Design review of the part built by this model. Coordinates are the model's own, in mm. A direction names the side the tool comes from. Round coordinates to 2 decimals unless told otherwise and drop trailing zeros. Order: outer loops, then holes, each group sorted by start corner. A loop starts at its lowest first (then second) coordinate and runs counter-clockwise, first axis right, second up. Notation, with made-up numbers: (-29.75, 74) - (-18.75, 74) arc R25 cw to (-18.75, 100) - close; hole circle Ø11 at (53.5, 49.25). An arc over 180 degrees is marked (long way). Answer as a JSON object with one key per item and string values. Group by question number.
from build123d import *

# Parameters (mm, degrees)
F0_R     = 2.13
F1_DEPTH = 5.5


# Not quite as in the source:
# - ends of sketch curves that miss each other by under 0.0002 mm in the source are joined


with BuildPart() as f1:
    # F0 (on Top) → F1 (new body)
    with BuildSketch(Plane.XY):
        with BuildLine():
            ThreePointArc((9.1999998704, 10.271), (8.8197324019, 8.3578320272), (7.735999997, 6.736000003))
            Line((7.735999997, 6.736000003), (-18.536, -19.536))
            ThreePointArc((-18.536, -19.536), (-20.1578320272, -20.6197324019), (-22.071, -20.9999998704))
            Line((-22.071, -20.9999998704), (-46, -21))
            ThreePointArc((-46, -21), (-49.5349996687, -22.4650003313), (-50.9999996674, -26.0000000001))
            Line((-50.9999996674, -26.0000000001), (-51, -37))
            ThreePointArc((-51, -37), (-49.5349996687, -40.5349996687), (-45.9999999999, -41.9999996674))
            Line((-45.9999999999, -41.9999996674), (46, -42))
            ThreePointArc((46, -42), (49.5349996687, -40.5349996687), (50.9999996674, -36.9999999999))
            Line((50.9999996674, -36.9999999999), (51, 37))
            ThreePointArc((51, 37), (49.5349996687, 40.5349996687), (45.9999999999, 41.9999996674))
            Line((45.9999999999, 41.9999996674), (14.2, 42))
            ThreePointArc((14.2, 42), (10.6650003313, 40.5349996687), (9.2000003326, 36.9999999999))
            Line((9.2000003326, 36.9999999999), (9.1999998704, 10.271))
        make_face()
        with Locations((-41.17, -33.07)):
            Circle(F0_R, mode=Mode.SUBTRACT)
        with Locations((-0.17, -33.07)):
            Circle(F0_R, mode=Mode.SUBTRACT)
        with Locations((41.17, -33.07)):
            Circle(F0_R, mode=Mode.SUBTRACT)
        with BuildLine():
            ThreePointArc((13, 4.6), (14.6, 6.2), (16.2, 4.6))
            Line((16.2, 4.6), (16.2, -1.4))
            ThreePointArc((16.2, -1.4), (14.6, -3), (13, -1.4))
            Line((13, -1.4), (13, 4.6))
        make_face(mode=Mode.SUBTRACT)
        with BuildLine():
            Line((47.2, 4.6), (47.2, -1.4))
            ThreePointArc((47.2, -1.4), (45.6, -3), (44, -1.4))
            Line((44, -1.4), (44, 4.6))
            ThreePointArc((44, 4.6), (45.6, 6.2), (47.2, 4.6))
        make_face(mode=Mode.SUBTRACT)
        with BuildLine():
            ThreePointArc((41.6, 14.3), (30.1, 2.8), (18.6, 14.3))
            Line((18.6, 14.3), (18.6, 20.3))
            ThreePointArc((18.6, 20.3), (30.1, 31.8), (41.6, 20.3))
            Line((41.6, 20.3), (41.6, 14.3))
        make_face(mode=Mode.SUBTRACT)
        with BuildLine():
            ThreePointArc((13, 35.6), (14.6, 37.2), (16.2, 35.6))
            Line((16.2, 35.6), (16.2, 29.6))
            ThreePointArc((16.2, 29.6), (14.6, 28), (13, 29.6))
            Line((13, 29.6), (13, 35.6))
        make_face(mode=Mode.SUBTRACT)
        with BuildLine():
            Line((47.2, 35.6), (47.2, 29.6))
            ThreePointArc((47.2, 29.6), (45.6, 28), (44, 29.6))
            Line((44, 29.6), (44, 35.6))
            ThreePointArc((44, 35.6), (45.6, 37.2), (47.2, 35.6))
        make_face(mode=Mode.SUBTRACT)
    extrude(amount=F1_DEPTH)


solid = f1.part
1. Take a section at A-A, the plane y = 0. Give the boundary of the cut face in (x, z), then the cut area to 3 significant figures.
2. Mouldability with a two-part tool opening along Y and no side actions: class faces 4 (the flat face through (11, -9, 5.5)), 5 (the cylindrical face through (-49, -22, 3)), 6 (the cylindrical face through (49, -41, 3)), 7 (the flat face through (44, 33, 3)) as pulls with the +Y half, pulls with the -Y half, needs draft (parallel to the pull), parting line crosses it, or undercut.
3. Take a section at D-D, the plane y = 9. Give the boundary of the cut face in (x, z), then the cut area to 3 significant figures.
4. To check wall thickness, follow line 1 (Y direction, x = 29.5, z = 2.4); line 2 (Y direction, x = -41.17, z = 2.7); line 3 (X direction, y = 6, z = 0.3). State the ranges of each line that lie inside material, in increasing order. Write a range as from..to.
5. Tool access review of faces 1 (the cylindrical face through (45.6, 6.2, 2.7)), 2 (the cylindrical face through (50, 40, 3)), 3 (the flat face through (-34, -21, 3)): name each direction out of +Z, -Z, +X, -X, +Y, -Y from which nothing blocks a thin tool from reaching the whole face with its end or side.
6. Clearance check with flat-ended pins moving along their axes: P1, Ø3.5, axis at x = 41.17, y = -33.07, coming from the +Z side; P2, Ø1.5, axis at x = -38.5, z = 1, coming from the +Y side; P3, Ø1.6, axis at y = 33.5, z = 3, coming from the -X side. State where each tip first meets the part, or that it passes through.
7. Take a section at C-C, the plane y = -33.07. Give the boundary of the cut face in (x, z), then the cut area to 3 significant figures.
8. Take a section at B-B, the plane x = -0.17. Give the boundary of the cut face in (y, z).
Response values:
{
 "1": {"outline": "(1, 0) - (13, 0) - (13, 5.5) - (1, 5.5) - close; (16.2, 0) - (44, 0) - (44, 5.5) - (16.2, 5.5) - close; (47.2, 0) - (51, 0) - (51, 5.5) - (47.2, 5.5) - close", "area": "240 mm2"},
 "2": {"face 4": "needs draft", "face 5": "pulls with the +Y half", "face 6": "pulls with the -Y half", "face 7": "undercut"},
 "3": {"outline": "(9.04, 0) - (19.89, 0) - (19.89, 5.5) - (9.04, 5.5) - close; (40.31, 0) - (51, 0) - (51, 5.5) - (40.31, 5.5) - close", "area": "119 mm2"},
 "4": {"line 1": "-42..2.82, 31.78..42", "line 2": "-42..-35.2, -30.94..-21", "line 3": "7..13.83, 15.37..22.14, 38.06..44.83, 46.37..51"},
 "5": {"face 1": "+Z, -Z", "face 2": "+Z, -Z, +X, +Y", "face 3": "+Z, -Z, -X, +Y"},
 "6": {"P1": "through", "P2": "y = -21", "P3": "x = 9.2"},
 "7": {"outline": "(-51, 0) - (-43.3, 0) - (-43.3, 5.5) - (-51, 5.5) - close; (-39.04, 0) - (-2.3, 0) - (-2.3, 5.5) - (-39.04, 5.5) - close; (1.96, 0) - (39.04, 0) - (39.04, 5.5) - (1.96, 5.5) - close; (43.3, 0) - (51, 0) - (51, 5.5) - (43.3, 5.5) - close", "area": "491 mm2"},
 "8": {"outline": "(-42, 0) - (-35.2, 0) - (-35.2, 5.5) - (-42, 5.5) - close; (-30.94, 0) - (-1.17, 0) - (-1.17, 5.5) - (-30.94, 5.5) - close"}
}
